from build123d import *

# Parameters (mm, degrees)
SKETCH1_R           = 3.75
BOSS_EXTRUDE1_DEPTH = 13
SKETCH2_R           = 5
BOSS_EXTRUDE2_DEPTH = 7
SKETCH3_R           = 2.85
CUT_EXTRUDE1_DEPTH  = 15
FILLET1_R           = 0.5
FILLET2_R           = 0.25
FILLET3_R           = 2


with BuildPart() as part:
    # Sketch1 → Boss-Extrude1 (new body)
    with BuildSketch(Plane.XY):
        with Locations(Location((0, 0, 0), (0, 0, 180))):
            Circle(SKETCH1_R)
    extrude(amount=BOSS_EXTRUDE1_DEPTH)

    # Sketch2 → Boss-Extrude2 (add)
    with BuildSketch(Plane.XY.offset(13)):
        Circle(SKETCH2_R)
    extrude(amount=BOSS_EXTRUDE2_DEPTH)

    # Sketch3 → Cut-Extrude1 (cut)
    with BuildSketch(Plane(origin=(0, 0, 0), x_dir=(-1, 0, 0), z_dir=(0, 0, -1))):
        Circle(SKETCH3_R)
    extrude(amount=-CUT_EXTRUDE1_DEPTH, mode=Mode.SUBTRACT)

    # Fillet1
    fillet1_edges = [part.edges().sort_by_distance(p)[0] for p in [
        (3.75, 0, 13),
        (-5, 0, 13),
    ]]
    fillet(fillet1_edges, radius=FILLET1_R)

    # Fillet2
    fillet2_edges = [part.edges().sort_by_distance(p)[0] for p in [
        (2.85, 0, 0),
        (3.75, 0, 0),
    ]]
    fillet(fillet2_edges, radius=FILLET2_R)

    # Fillet3
    fillet3_edges = [part.edges().sort_by_distance(p)[0] for p in [
        (-5, 0, 20),
    ]]
    fillet(fillet3_edges, radius=FILLET3_R)


solid = part.part
Source: CAD feature listing. Evaluate the final solid. Frame: model axes, mm. Give positions to 0.01 mm unless a question says otherwise; leave off trailing zeros. Order: outer loops, then holes, each group sorted by start corner. A loop starts at its lowest first (then second) coordinate and runs counter-clockwise, first axis right, second up. Notation, with made-up numbers: (37.25, 19) -> (71.25, 19) arc R19 ccw to (71.25, 33) -> close; hole circle Ø2 at (-24, 15.5). An arc over 180 degrees is marked (long way). Write item = value, one per line.
Q1. Cut plane A-A, the plane y = 0. Output: boundary loops of the cut face in (x, z).
Data:
outline = (-5, 13.5) arc R0.5 ccw to (-4.5, 13) -> (-4.25, 13) arc R0.5 cw to (-3.75, 12.5) -> (-3.75, 0.25) arc R0.25 ccw to (-3.5, 0) -> (-3.1, 0) arc R0.25 ccw to (-2.85, 0.25) -> (-2.85, 15) -> (2.85, 15) -> (2.85, 0.25) arc R0.25 ccw to (3.1, 0) -> (3.5, 0) arc R0.25 ccw to (3.75, 0.25) -> (3.75, 12.5) arc R0.5 cw to (4.25, 13) -> (4.5, 13) arc R0.5 ccw to (5, 13.5) -> (5, 18) arc R2 ccw to (3, 20) -> (-3, 20) arc R2 ccw to (-5, 18) -> close
Q2. Pull-direction query (Y, two-part tool) for faces 1 (the face through (0, 0, 20)), 2 (the face through (2.262, -1.734, 7.522)), 3 (the face through (-1.08, -4.88, 15.72)); classes: released by +Y, released by -Y, zero draft, split by the parting line, or undercut.
Data:
face_1 = zero draft
face_2 = undercut
face_3 = split by the parting line
Q3. Pin query (flat end, axial travel): pin 1 (3 mm diameter, centred on x = -1.5, y = 0, fed in from -Z); pin 2 (4.5 mm diameter, centred on x = 0, y = 0, fed in from -Z); pin 3 (4 mm diameter, centred on x = 0.5, z = 6, fed in from +Y). Return the tip coordinate at first contact, or that it passes through.
Data:
pin_1 = 0.02
pin_2 = 15
pin_3 = 3.75
Q4. Material intervals for line 1 (Y direction, x = 0, z = 4); line 2 (Z direction, x = -1.5, y = 1.25); line 3 (Y direction, x = -1.5, z = 5), sorted ascending. Write a range as from..to.
Data:
line_1 = -3.75..-2.85, 2.85..3.75
line_2 = 15..20
line_3 = -3.44..-2.42, 2.42..3.44
Q5. Cut plane D-D, the plane z = 12.25. Output: boundary loops of the cut face in (x, y).
Data:
outline = circle Ø7.5 at (0, 0); hole circle Ø5.7 at (0, 0)
Q6. Cut plane B-B, the plane z = 14.5. Output: boundary loops of the cut face in (x, y).
Data:
outline = circle Ø10 at (0, 0); hole circle Ø5.7 at (0, 0)
